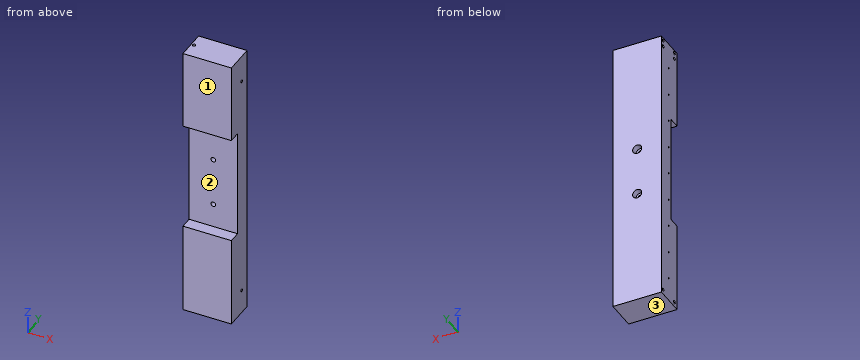
```python
from build123d import *

# Parameters (mm, degrees)
SKETCH1_W           = 101.6
SKETCH1_H           = 63.5
BOSS_EXTRUDE1_DEPTH = 585.0001
SKETCH2_W           = 228.6
SKETCH2_H           = 25
CUT_EXTRUDE1_DEPTH  = 102.6
SKETCH5_R           = 1.75
CUT_EXTRUDE4_DEPTH  = 6.35
SKETCH5_3_R         = 3.3
CUT_EXTRUDE5_DEPTH  = 25.4
SKETCH6_R           = 4.934351916
CUT_EXTRUDE6_DEPTH  = 39.5
CUT_EXTRUDE7_DEPTH  = 12.7
SKETCH8_R           = 3.175
CUT_EXTRUDE8_DEPTH  = 12.7
CUT_EXTRUDE9_START  = 50.8
SKETCH9_R           = 9.525
CUT_EXTRUDE9_DEPTH  = 14.1


with BuildPart() as part:
    # Sketch1 → Boss-Extrude1 (new body)
    with BuildSketch(Plane.XY):
        with Locations((50.8, 31.75)):
            Rectangle(SKETCH1_W, SKETCH1_H)
    extrude(amount=BOSS_EXTRUDE1_DEPTH)

    # Sketch2 → Cut-Extrude1 (cut, through all)
    with BuildSketch(Plane.ZY):
        with Locations((304.8, 12.5)):
            Rectangle(SKETCH2_W, SKETCH2_H)
    extrude(amount=-CUT_EXTRUDE1_DEPTH, mode=Mode.SUBTRACT)

    # Sketch5 → Cut-Extrude4 (cut)
    with BuildSketch(Plane.ZY):
        with Locations((530, 33.5)):
            Circle(SKETCH5_R)
        with Locations((470, 33.5)):
            Circle(SKETCH5_R)
        with Locations((410, 33.5)):
            Circle(SKETCH5_R)
        with Locations((350, 33.5)):
            Circle(SKETCH5_R)
        with Locations((290, 33.5)):
            Circle(SKETCH5_R)
        with Locations((230, 33.5)):
            Circle(SKETCH5_R)
        with Locations((170, 33.5)):
            Circle(SKETCH5_R)
        with Locations((110, 33.5)):
            Circle(SKETCH5_R)
        with Locations((50, 33.5)):
            Circle(SKETCH5_R)
    extrude(amount=-CUT_EXTRUDE4_DEPTH, mode=Mode.SUBTRACT)

    # Sketch5_3 → Cut-Extrude5 (cut)
    with BuildSketch(Plane.ZY):
        with Locations((579, 10.5)):
            Circle(SKETCH5_3_R)
        with Locations((566, 10.5)):
            Circle(SKETCH5_3_R)
        with Locations((579, 56.5)):
            Circle(SKETCH5_3_R)
        with Locations((566, 56.5)):
            Circle(SKETCH5_3_R)
        with Locations((10, 10.5)):
            Circle(SKETCH5_3_R)
        with Locations((10, 56.5)):
            Circle(SKETCH5_3_R)
    extrude(amount=-CUT_EXTRUDE5_DEPTH, mode=Mode.SUBTRACT)

    # Sketch6 → Cut-Extrude6 (cut, through all)
    with BuildSketch(Plane.XZ.offset(-25)):
        with Locations((50.8, 342.9)):
            Circle(SKETCH6_R)
        with Locations((50.8, 241.3)):
            Circle(SKETCH6_R)
    extrude(amount=-CUT_EXTRUDE6_DEPTH, mode=Mode.SUBTRACT)

    # Sketch7 → Cut-Extrude7 (cut)
    with BuildSketch(Plane(origin=(101.6, 0, 0), x_dir=(0, 0, -1), z_dir=(1, 0, 0))):
        with BuildLine():
            ThreePointArc((-53.548542941, 39.694194493), (-50.80220266, 38.11238), (-48.055862379, 39.694194493))
            ThreePointArc((-48.055862379, 39.694194493), (-47.62720266, 41.28738), (-48.055862379, 42.880565507))
            ThreePointArc((-48.055862379, 42.880565507), (-50.80220266, 44.46238), (-53.548542941, 42.880565507))
            ThreePointArc((-53.548542941, 42.880565507), (-53.97720266, 41.28738), (-53.548542941, 39.694194493))
        make_face()
        with BuildLine():
            ThreePointArc((-525.637642589, 39.694194493), (-525.20898287, 41.28738), (-525.637642589, 42.880565507))
            ThreePointArc((-525.637642589, 42.880565507), (-528.38398287, 44.46238), (-531.130323151, 42.880565507))
            ThreePointArc((-531.130323151, 42.880565507), (-531.55898287, 41.28738), (-531.130323151, 39.694194493))
            ThreePointArc((-531.130323151, 39.694194493), (-528.38398287, 38.11238), (-525.637642589, 39.694194493))
        make_face()
    extrude(amount=-CUT_EXTRUDE7_DEPTH, mode=Mode.SUBTRACT)

    # Sketch8 → Cut-Extrude8 (cut)
    with BuildSketch(Plane.XY.offset(585.0001)):
        with Locations((5.95, 33.5)):
            Circle(SKETCH8_R)
    extrude(amount=-CUT_EXTRUDE8_DEPTH, mode=Mode.SUBTRACT)

    # Sketch9 → Cut-Extrude9 (cut, through all)
    with BuildSketch(Plane(origin=(0, -0.4, 0), x_dir=(1, 0, 0), z_dir=(0, 1, 0)).offset(CUT_EXTRUDE9_START)):
        with Locations((50.8, -342.9)):
            Circle(SKETCH9_R)
        with Locations((50.8, -241.3)):
            Circle(SKETCH9_R)
    extrude(amount=CUT_EXTRUDE9_DEPTH, mode=Mode.SUBTRACT)


solid = part.part
```
Geometry check sheet. Reference: the model listing, model coordinates, mm. Face numbers are marked on the shaded views. Give positions to 0.01 mm unless a question says otherwise; leave off trailing zeros. Order: outer loops, then holes, each group sorted by start corner. A loop starts at its lowest first (then second) coordinate and runs counter-clockwise, first axis right, second up. Notation, with made-up numbers: (-18.75, 12) -> (25.25, 12) arc R29 cw to (25.25, 32) -> close; hole circle Ø6 at (21, -7.75). An arc over 180 degrees is marked (long way). Write each question's results on one line, items separated by ' | '. Start each with the question number.
(1) Sectioned sample at B-B (x = 30.5). Enter the section's corners in (y, z).
(2) Scan lines: line 1 (Z direction, x = 50.8, y = 41.75); line 2 (Y direction, x = 11.25, z = 579); line 3 (X direction, y = 33, z = 581). Record each from-to range of solid material in increasing order.
(3) Gauge pin test, flat ends, axial feed: P1, Ø5.5, axis at x = 5.95, y = 33.5, coming from the +Z side; P2, Ø1, axis at y = 32.5, z = 230, coming from the -X side; P3, Ø6, axis at x = 56, z = 236.5, coming from the -Y side. Record the tip position at first contact, or that the pin passes through.
(4) Mould release check, pull along Z, two halves, no side actions. Record for the marked faces 1, 2 and 3: pulls with the +Z half, pulls with the -Z half, needs draft (parallel to the pull), parting line crosses it, or undercut.
(5) Sectioned sample at A-A (z = 241.3). Enter the section's corners in (x, y) (3 decimals), plus the area to 3 significant figures.
Answer below:
1) outline: (0, 0) -> (63.5, 0) -> (63.5, 585) -> (0, 585) -> (0, 419.1) -> (25, 419.1) -> (25, 190.5) -> (0, 190.5) -> close
2) line 1: 0 to 236.37, 246.23 to 337.97, 347.83 to 585 | line 2: 0 to 7.2, 13.8 to 53.2, 59.8 to 63.5 | line 3: 0 to 2.81, 9.09 to 101.6
3) P1: z = 572.3 | P2: x = 6.35 | P3: y = 25
4) face 1: needs draft | face 2: undercut | face 3: pulls with the -Z half
5) outline: (0, 25) -> (45.866, 25) -> (45.866, 50.4) -> (41.275, 50.4) -> (41.275, 63.5) -> (0, 63.5) -> close; (55.734, 25) -> (101.6, 25) -> (101.6, 63.5) -> (60.325, 63.5) -> (60.325, 50.4) -> (55.734, 50.4) -> close | area: 3,410 mm2
